from build123d import *

# Parameters (mm, degrees)
SKETCH_1_R          = 2.25
EXTRUDE_1_DEPTH     = 30.25
CUT_EXTRUDE_1_DEPTH = 26.6
CUT_EXTRUDE_2_DEPTH = 2.5


with BuildPart() as part:
    # 草圖1 → 填料-伸長1 (new body)
    with BuildSketch(Plane(origin=(0, 0, 0), x_dir=(1, 0, 0), z_dir=(0, 1, 0))):
        with BuildLine():
            Line((6.340909091, 120.340909091), (114.340909091, 120.340909091))
            ThreePointArc((114.340909091, 120.340909091), (118.583549778, 118.583549778), (120.340909091, 114.340909091))
            Line((120.340909091, 114.340909091), (120.340909091, 6.340909091))
            ThreePointArc((120.340909091, 6.340909091), (118.583549778, 2.098268404), (114.340909091, 0.340909091))
            Line((114.340909091, 0.340909091), (6.340909091, 0.340909091))
            ThreePointArc((6.340909091, 0.340909091), (2.098268404, 2.098268404), (0.340909091, 6.340909091))
            Line((0.340909091, 6.340909091), (0.340909091, 114.340909091))
            ThreePointArc((0.340909091, 114.340909091), (2.098268404, 118.583549778), (6.340909091, 120.340909091))
        make_face()
        with Locations(Location((7.340909091, 113.340909091, 0), (0, 0, 270))):
            Circle(SKETCH_1_R, mode=Mode.SUBTRACT)
        with Locations(Location((113.340909091, 113.340909091, 0), (0, 0, 270))):
            Circle(SKETCH_1_R, mode=Mode.SUBTRACT)
        with Locations(Location((7.340909091, 7.340909091, 0), (0, 0, 270))):
            Circle(SKETCH_1_R, mode=Mode.SUBTRACT)
        with Locations(Location((113.340909091, 7.340909091, 0), (0, 0, 270))):
            Circle(SKETCH_1_R, mode=Mode.SUBTRACT)
    extrude(amount=EXTRUDE_1_DEPTH)

    # 草圖2 → 除料-伸長1 (cut)
    with BuildSketch(Plane(origin=(0, 30.25, 0), x_dir=(1, 0, 0), z_dir=(0, 1, 0))):
        with BuildLine():
            Line((15.940908992, 101.053812481), (15.940908992, 107.840909091))
            Line((15.940908992, 107.840909091), (1.440909091, 107.840909091))
            Line((1.440909091, 107.840909091), (1.440909091, 96.184307649))
            ThreePointArc((1.440909091, 96.184307649), (1.788763936, 95.708017977), (2.348316498, 95.894446985))
            ThreePointArc((2.348316498, 95.894446985), (4.094702185, 97.408643653), (6.340909091, 97.953812481))
            Line((6.340909091, 97.953812481), (12.840908992, 97.953812481))
            ThreePointArc((12.840908992, 97.953812481), (15.032940014, 98.861781459), (15.940908992, 101.053812481))
        make_face()
        with BuildLine():
            Line((6.328095563, 22.75810538), (12.727920948, 22.741369743))
            ThreePointArc((12.727920948, 22.741369743), (14.940810853, 21.804058056), (15.818922369, 19.567016463))
            Line((15.818922369, 19.567016463), (15.65752772, 12.840909091))
            Line((15.65752772, 12.840909091), (1.440909091, 12.840909091))
            Line((1.440909091, 12.840909091), (1.440909091, 24.527593458))
            ThreePointArc((1.440909091, 24.527593458), (1.788763936, 25.00388313), (2.348316498, 24.817454121))
            ThreePointArc((2.348316498, 24.817454121), (4.089010146, 23.306198101), (6.328095563, 22.75810538))
        make_face()
        with BuildLine():
            Line((99.84090919, 115.840909091), (20.840908992, 115.840909091))
            ThreePointArc((20.840908992, 115.840909091), (19.78024882, 115.401569263), (19.340908992, 114.340909091))
            Line((19.340908992, 114.340909091), (19.340908992, 101.053812481))
            ThreePointArc((19.340908992, 101.053812481), (17.43710307, 96.457618403), (12.840908992, 94.553812481))
            Line((12.840908992, 94.553812481), (6.340909091, 94.553812481))
            ThreePointArc((6.340909091, 94.553812481), (5.280248919, 94.114472652), (4.840909091, 93.053812481))
            Line((4.840909091, 93.053812481), (4.840909091, 27.658088626))
            ThreePointArc((4.840909091, 27.658088626), (5.278863008, 26.598816178), (6.336986582, 26.158093755))
            Line((6.336986582, 26.158093755), (12.736811967, 26.141358118))
            ThreePointArc((12.736811967, 26.141358118), (17.376742412, 24.176027162), (19.217943979, 19.485456079))
            Line((19.217943979, 19.485456079), (18.903400656, 6.376891613))
            ThreePointArc((18.903400656, 6.376891613), (19.32966249, 5.293047884), (20.402969013, 4.840909091))
            Line((20.402969013, 4.840909091), (99.84090919, 4.840909091))
            ThreePointArc((99.84090919, 4.840909091), (100.901569362, 5.280248919), (101.34090919, 6.340909091))
            Line((101.34090919, 6.340909091), (101.34090919, 19.628005701))
            ThreePointArc((101.34090919, 19.628005701), (103.244715112, 24.224199779), (107.84090919, 26.128005701))
            Line((107.84090919, 26.128005701), (114.340909091, 26.128005701))
            ThreePointArc((114.340909091, 26.128005701), (115.401569263, 26.567345529), (115.840909091, 27.628005701))
            Line((115.840909091, 27.628005701), (115.840909091, 93.053812481))
            ThreePointArc((115.840909091, 93.053812481), (115.401569263, 94.114472652), (114.340909091, 94.553812481))
            Line((114.340909091, 94.553812481), (107.84090919, 94.553812481))
            ThreePointArc((107.84090919, 94.553812481), (103.244715112, 96.457618403), (101.34090919, 101.053812481))
            Line((101.34090919, 101.053812481), (101.34090919, 114.340909091))
            ThreePointArc((101.34090919, 114.340909091), (100.901569362, 115.401569263), (99.84090919, 115.840909091))
        make_face()
        with BuildLine():
            Line((104.74090919, 19.628005701), (104.74090919, 12.840909091))
            Line((104.74090919, 12.840909091), (119.240909091, 12.840909091))
            Line((119.240909091, 12.840909091), (119.240909091, 24.497510533))
            ThreePointArc((119.240909091, 24.497510533), (118.893054246, 24.973800205), (118.333501683, 24.787371196))
            ThreePointArc((118.333501683, 24.787371196), (116.587115997, 23.273174529), (114.340909091, 22.728005701))
            Line((114.340909091, 22.728005701), (107.84090919, 22.728005701))
            ThreePointArc((107.84090919, 22.728005701), (105.648878168, 21.820036723), (104.74090919, 19.628005701))
        make_face()
        with BuildLine():
            Line((114.340909091, 97.953812481), (107.84090919, 97.953812481))
            ThreePointArc((107.84090919, 97.953812481), (105.648878168, 98.861781459), (104.74090919, 101.053812481))
            Line((104.74090919, 101.053812481), (104.74090919, 107.840909091))
            Line((104.74090919, 107.840909091), (119.240909091, 107.840909091))
            Line((119.240909091, 107.840909091), (119.240909091, 96.184307649))
            ThreePointArc((119.240909091, 96.184307649), (118.893054246, 95.708017977), (118.333501683, 95.894446985))
            ThreePointArc((118.333501683, 95.894446985), (116.587115997, 97.408643653), (114.340909091, 97.953812481))
        make_face()
    extrude(amount=-CUT_EXTRUDE_1_DEPTH, mode=Mode.SUBTRACT)

    # 草圖3 → 除料-伸長2 (cut)
    with BuildSketch(Plane(origin=(0, 30.25, 0), x_dir=(1, 0, 0), z_dir=(0, 1, 0))):
        with BuildLine():
            Line((103.84090919, 101.053812481), (103.84090919, 114.340909091))
            ThreePointArc((103.84090919, 114.340909091), (102.669336315, 117.169336216), (99.84090919, 118.340909091))
            Line((99.84090919, 118.340909091), (20.840908992, 118.340909091))
            ThreePointArc((20.840908992, 118.340909091), (18.012481867, 117.169336216), (16.840908992, 114.340909091))
            Line((16.840908992, 114.340909091), (16.840908992, 101.053812481))
            ThreePointArc((16.840908992, 101.053812481), (15.669336117, 98.225385356), (12.840908992, 97.053812481))
            Line((12.840908992, 97.053812481), (6.340909091, 97.053812481))
            ThreePointArc((6.340909091, 97.053812481), (3.512481966, 95.882239605), (2.340909091, 93.053812481))
            Line((2.340909091, 93.053812481), (2.340909091, 27.658088626))
            ThreePointArc((2.340909091, 27.658088626), (3.508786204, 24.833362099), (6.330449068, 23.658102303))
            Line((6.330449068, 23.658102303), (12.730274453, 23.641366666))
            ThreePointArc((12.730274453, 23.641366666), (15.585616265, 22.431932231), (16.718663383, 19.545426949))
            Line((16.718663383, 19.545426949), (16.40412006, 6.436862484))
            ThreePointArc((16.40412006, 6.436862484), (17.540818286, 3.54661254), (20.402969013, 2.340909091))
            Line((20.402969013, 2.340909091), (99.84090919, 2.340909091))
            ThreePointArc((99.84090919, 2.340909091), (102.669336315, 3.512481966), (103.84090919, 6.340909091))
            Line((103.84090919, 6.340909091), (103.84090919, 19.628005701))
            ThreePointArc((103.84090919, 19.628005701), (105.012482065, 22.456432826), (107.84090919, 23.628005701))
            Line((107.84090919, 23.628005701), (114.340909091, 23.628005701))
            ThreePointArc((114.340909091, 23.628005701), (117.169336216, 24.799578576), (118.340909091, 27.628005701))
            Line((118.340909091, 27.628005701), (118.340909091, 93.053812481))
            ThreePointArc((118.340909091, 93.053812481), (117.169336216, 95.882239605), (114.340909091, 97.053812481))
            Line((114.340909091, 97.053812481), (107.84090919, 97.053812481))
            ThreePointArc((107.84090919, 97.053812481), (105.012482065, 98.225385356), (103.84090919, 101.053812481))
        make_face()
        with BuildLine():
            Line((114.340909091, 95.453812481), (107.84090919, 95.453812481))
            ThreePointArc((107.84090919, 95.453812481), (103.881111215, 97.094014506), (102.24090919, 101.053812481))
            Line((102.24090919, 101.053812481), (102.24090919, 114.340909091))
            ThreePointArc((102.24090919, 114.340909091), (101.537965465, 116.037965366), (99.84090919, 116.740909091))
            Line((99.84090919, 116.740909091), (20.840908992, 116.740909091))
            ThreePointArc((20.840908992, 116.740909091), (19.143852717, 116.037965366), (18.440908992, 114.340909091))
            Line((18.440908992, 114.340909091), (18.440908992, 101.053812481))
            ThreePointArc((18.440908992, 101.053812481), (16.800706967, 97.094014506), (12.840908992, 95.453812481))
            Line((12.840908992, 95.453812481), (6.340909091, 95.453812481))
            ThreePointArc((6.340909091, 95.453812481), (4.643852816, 94.750868756), (3.940909091, 93.053812481))
            Line((3.940909091, 93.053812481), (3.940909091, 27.658088626))
            ThreePointArc((3.940909091, 27.658088626), (4.641635359, 25.96325271), (6.334633077, 25.258096832))
            Line((6.334633077, 25.258096832), (12.734458462, 25.241361195))
            ThreePointArc((12.734458462, 25.241361195), (16.731936999, 23.548152987), (18.318202964, 19.507045592))
            Line((18.318202964, 19.507045592), (18.003659641, 6.398481127))
            ThreePointArc((18.003659641, 6.398481127), (18.685678577, 4.66433116), (20.402969013, 3.940909091))
            Line((20.402969013, 3.940909091), (99.84090919, 3.940909091))
            ThreePointArc((99.84090919, 3.940909091), (101.537965465, 4.643852816), (102.24090919, 6.340909091))
            Line((102.24090919, 6.340909091), (102.24090919, 19.628005701))
            ThreePointArc((102.24090919, 19.628005701), (103.881111215, 23.587803676), (107.84090919, 25.228005701))
            Line((107.84090919, 25.228005701), (114.340909091, 25.228005701))
            ThreePointArc((114.340909091, 25.228005701), (116.037965366, 25.930949426), (116.740909091, 27.628005701))
            Line((116.740909091, 27.628005701), (116.740909091, 93.053812481))
            ThreePointArc((116.740909091, 93.053812481), (116.037965366, 94.750868756), (114.340909091, 95.453812481))
        make_face(mode=Mode.SUBTRACT)
    extrude(amount=-CUT_EXTRUDE_2_DEPTH, mode=Mode.SUBTRACT)


solid = part.part
Part model, mm, in its own coordinate system. A direction names the side the tool comes from. Give positions to 0.01 mm unless a question says otherwise; leave off trailing zeros. Loops run counter-clockwise (first coordinate to the right, second up) from the corner with the lowest first, then second, coordinate; pieces in that order, holes last. Notation, with made-up numbers: M -1,8.5 L 58,8.5 A25 ccw 58,43.5 Z; hole C 78.25,13 d7. An arc over 180 degrees is marked long. Put each result on its own line as item: value. Start each with the question number.
1) Saw through at B-B (z = -49.5). List the corners of the cut face in (x, y), then the cut area to 3 significant figures.
2) Probe probe 1 along X at (y, z) = (12.5, -20); probe 2 along Z at (x, y) = (23, 11); probe 3 along X at (y, z) = (17, -86.5). List the from-to ranges inside material, lowest first.
3) Flat gauge pin, fed straight in: pin 1 (6 mm diameter, centred on x = 83, z = -66.5, fed in from +Y). Where does the tip first touch, or does it go through?
4) 3-axis set-ups, long thin cutter, end or side, ignore diameter. For faces 1 (the flat face through (17, 27.75, -22)), 2 (the cylindrical face through (7.44, 14.91, -115.59)): which of +Z, -Z, +X, -X, +Y, -Y reach the whole face in a straight line?
5) Saw through at C-C (z = -15.5). List the corners of the cut face in (x, y).
6) Saw through at A-A (x = 37). List the corners of the cut face in (y, z).
7) Saw through at D-D (y = 26). State how many separate pieces and enclosed holes the cut face has, then the cut area to 3 significant figures.
Numbers:
1. outline: M 0.34,0 L 120.34,0 L 120.34,30.25 L 118.34,30.25 L 118.34,27.75 L 116.74,27.75 L 116.74,30.25 L 115.84,30.25 L 115.84,3.65 L 4.84,3.65 L 4.84,30.25 L 3.94,30.25 L 3.94,27.75 L 2.34,27.75 L 2.34,30.25 L 0.34,30.25 Z
1. area: 669 mm^2
2. probe 1: 0.34 to 1.44, 15.8 to 19.21, 101.35 to 104.76, 119.24 to 120.34
2. probe 2: -120.34 to -115.84, -4.84 to -0.34
2. probe 3: 0.34 to 4.84, 115.84 to 120.34
3. pin 1: y = 3.65
4. face 1: +Y
4. face 2: +Y, -Y
5. outline: M 0.34,0 L 120.34,0 L 120.34,30.25 L 119.24,30.25 L 119.24,3.65 L 104.74,3.65 L 104.74,30.25 L 103.84,30.25 L 103.84,27.75 L 102.24,27.75 L 102.24,30.25 L 101.34,30.25 L 101.34,3.65 L 19.12,3.65 L 19.12,30.25 L 18.22,30.25 L 18.22,27.75 L 16.62,27.75 L 16.62,30.25 L 15.72,30.25 L 15.72,3.65 L 1.44,3.65 L 1.44,30.25 L 0.34,30.25 Z
6. outline: M 0,-120.34 L 30.25,-120.34 L 30.25,-118.34 L 27.75,-118.34 L 27.75,-116.74 L 30.25,-116.74 L 30.25,-115.84 L 3.65,-115.84 L 3.65,-4.84 L 30.25,-4.84 L 30.25,-3.94 L 27.75,-3.94 L 27.75,-2.34 L 30.25,-2.34 L 30.25,-0.34 L 0,-0.34 Z
7. separate pieces: 1
7. enclosed holes: 9
7. area: 2,600 mm^2
